```python
from build123d import *

# Parameters (mm, degrees)
F0_W      = 30
F0_H      = 30
F1_DEPTH  = 30
F2_W      = 10
F2_H      = 30
F3_DEPTH  = 0.5
F4_W      = 30
F4_H      = 10
F5_DEPTH  = 0.5
F6_W      = 30
F6_H      = 10
F7_DEPTH  = 0.5
F8_W      = 10
F8_H      = 30
F9_DEPTH  = 0.5
F11_DEPTH = 0.5
F13_DEPTH = 0.5


with BuildPart() as f1:
    # F0 (on Top) → F1 (new body)
    with BuildSketch(Plane.XY):
        with Locations((15, -15)):
            Rectangle(F0_W, F0_H)
    extrude(amount=F1_DEPTH)

    # F2 (on face) → F3 (join)
    with BuildSketch(Plane.XY.offset(30)):
        with Locations((15, -15)):
            Rectangle(F2_W, F2_H)
    extrude(amount=F3_DEPTH)

    # F4 (on face) → F5 (join)
    with BuildSketch(Plane(origin=(0, 0, 0), x_dir=(0, -1, 0), z_dir=(-1, 0, 0))):
        with Locations((15, 15)):
            Rectangle(F4_W, F4_H)
    extrude(amount=F5_DEPTH)

    # F6 (on face) → F7 (join)
    with BuildSketch(Plane.YZ.offset(30)):
        with Locations((-15, 15)):
            Rectangle(F6_W, F6_H)
    extrude(amount=F7_DEPTH)

    # F8 (on face) → F9 (join)
    with BuildSketch(Plane(origin=(0, 0, 0), x_dir=(1, 0, 0), z_dir=(0, 0, -1))):
        with Locations((15, 15)):
            Rectangle(F8_W, F8_H)
    extrude(amount=F9_DEPTH)

    # F10 (on face) → F11 (join)
    with BuildSketch(Plane.XZ.offset(30)):
        Polygon((10, -0.5), (20, -0.5), (20, 0), (20, 10), (30, 10), (30.5, 10), (30.5, 20), (30, 20), (20, 20), (20, 30), (20, 30.5), (10, 30.5), (10, 30), (10, 20), (0, 20), (-0.5, 20), (-0.5, 10), (0, 10), (10, 10), (10, 0), align=None)
    extrude(amount=F11_DEPTH)

    # F12 (on face) → F13 (join)
    with BuildSketch(Plane(origin=(0, 0, 0), x_dir=(-1, 0, 0), z_dir=(0, 1, 0))):
        Polygon((-20, 10), (-20, -0.5), (-10, -0.5), (-10, 10), (0.5, 10), (0.5, 20), (-10, 20), (-10, 30.5), (-20, 30.5), (-20, 20), (-30.5, 20), (-30.5, 10), align=None)
    extrude(amount=F13_DEPTH)


solid = f1.part
```
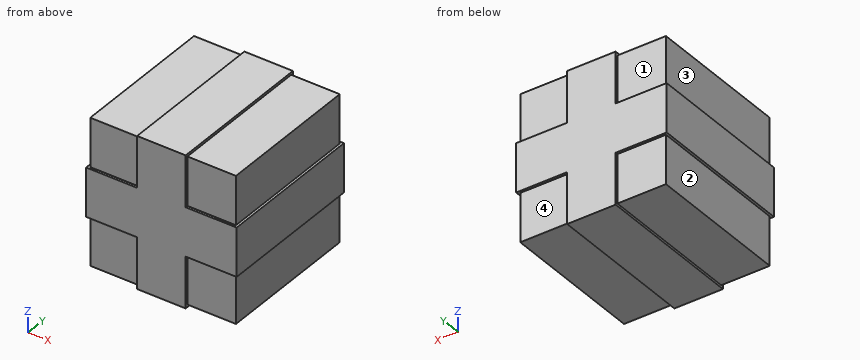
The model under review builds one solid part; all positions refer to its coordinate system, in mm. Face numbers are marked on the shaded views. A direction names the side the tool comes from. Coordinates: 2 decimals unless noted, no trailing zeros. Order: outer loops, then holes, each group sorted by start corner. A loop starts at its lowest first (then second) coordinate and runs counter-clockwise, first axis right, second up. Notation, with made-up numbers: M 73,39 L 103,39 A13 cw 103,50 Z; hole C 46.25,18.5 d7. An arc over 180 degrees is marked long. One line per question, with ' | ' between items.
(1) For probe 1 along X at (y, z) = (-27, 2); probe 2 along Y at (x, z) = (6.5, 4), list the stretches that pass through material, from the lowest coordinate up. Write a range as from..to.
Geometry results:
probe 1: x = 0..30 | probe 2: y = -30..0
(2) Machinability: for the marked faces 1, 2, 3 and 4, which of the approach directions +Z, -Z, +X, -X, +Y, -Y give a long, thin tool a straight path to every point of the face, cutting with its end or side? Answer none if there is none.
Geometry results:
face 1: +Z, -X, +Y | face 2: -Z, -X, +Y, -Y | face 3: +Z, -X, +Y, -Y | face 4: -Z, +X, +Y
(3) Insertion check: pin 1 (3 mm diameter, centred on x = 25, y = -16, fed in from +Z); pin 2 (8 mm diameter, centred on x = 7, z = 22.5, fed in from -Y); pin 3 (1.5 mm diameter, centred on x = 5, z = 5, fed in from +Y); pin 4 (3 mm diameter, centred on y = -19.5, z = 7.5, fed in from +X). Each pin has a flat end and moves straight along its axis. Give the tip position at first contact, or say it passes through.
Geometry results:
pin 1: stops at z = 30 | pin 2: stops at y = -30.5 | pin 3: stops at y = 0 | pin 4: stops at x = 30
(4) Add section B-B, the plane x = 20.5. Write out the cut boundary in (y, z), then the cut area to 3 significant figures.
Geometry results:
outline: M -30.5,10 L -30,10 L -30,0 L 0,0 L 0,10 L 0.5,10 L 0.5,20 L 0,20 L 0,30 L -30,30 L -30,20 L -30.5,20 Z | area: 910 mm²
(5) Add section A-A, the plane z = 26. Write out the cut boundary in (x, y), then the cut area to 3 significant figures.
Geometry results:
outline: M 0,-30 L 10,-30 L 10,-30.5 L 20,-30.5 L 20,-30 L 30,-30 L 30,0 L 20,0 L 20,0.5 L 10,0.5 L 10,0 L 0,0 Z | area: 910 mm²
(6) Add section C-C, the plane y = -19. Write out the cut boundary in (x, z), then the cut area to 3 significant figures.
Geometry results:
outline: M -0.5,10 L 0,10 L 0,0 L 10,0 L 10,-0.5 L 20,-0.5 L 20,0 L 30,0 L 30,10 L 30.5,10 L 30.5,20 L 30,20 L 30,30 L 20,30 L 20,30.5 L 10,30.5 L 10,30 L 0,30 L 0,20 L -0.5,20 Z | area: 920 mm²
